from build123d import *

# Parameters (mm, degrees)
SKETCH_1_R              = 12
EXTRUDE_1_DEPTH         = 12
DELETE_BODY_1_OUTLINE_R = 5
DELETE_BODY_1_DEPTH     = 12
EXTRUDE_START           = -1
SKETCH_2_R              = 12
EXTRUDE_2_DEPTH         = 1
SKETCH_3_W              = 2
SKETCH_3_H              = 13
SKETCH_5_W              = 34.262916627
SKETCH_5_H              = 20.154656839
CUT_EXTRUDE_3_DEPTH     = 24.151673806
SKETCH_6_R              = 1.25
EXTRUDE_4_DEPTH         = 2
SKETCH_7_R              = 4
EXTRUDE_5_DEPTH         = 2


# Read off the part's stored shape, not the designer's step: the other step, the delete body step
with BuildPart() as part:
    # Sketch 1 → Extrude 1 (new body)
    with BuildSketch(Plane.XY):
        Circle(SKETCH_1_R)
    extrude(amount=EXTRUDE_1_DEPTH)

    # Other 1 outline → Other 1 (revolve, cut)
    with BuildSketch(Plane.XZ):
        with BuildLine():
            Line((12, 12), (4, 12))
            Line((4, 12), (4, 8))
            Line((4, 8), (5, 8))
            Line((5, 8), (5, 4))
            Line((5, 4), (4, 4))
            Line((4, 4), (4, 0))
            Line((4, 0), (12, 0))
            Line((12, 0), (12, 1))
            ThreePointArc((12, 1), (7, 6), (12, 11))
            Line((12, 11), (12, 12))
        make_face()
    revolve(axis=Axis((0, 0, 0), (0, 0, 1)), mode=Mode.SUBTRACT)

    # Delete Body 1 outline → Delete Body 1 (cut)
    with BuildSketch(Plane.XY):
        Circle(DELETE_BODY_1_OUTLINE_R)
    extrude(amount=DELETE_BODY_1_DEPTH, mode=Mode.SUBTRACT)



with BuildPart() as body_2:
    # Sketch 2 → Extrude 2 (new body)
    with BuildSketch(Plane.XY.offset(EXTRUDE_START)):
        with Locations(Location((0, 0, 0), (0, 0, 270))):
            Circle(SKETCH_2_R)
    extrude(amount=EXTRUDE_2_DEPTH)


with BuildPart() as part_1:
    add(part.part)

    add(body_2.part)  # Revolve 1 merges body 2
    # Sketch 3 → Revolve 1 (revolve)
    with BuildSketch(Plane(origin=(0, 0, 0), x_dir=(1, 0, 0), z_dir=(0, 1, 0))):
        with Locations((-13, -5.5)):
            Rectangle(SKETCH_3_W, SKETCH_3_H)
    revolve(axis=Axis((0, 0, 0), (0, 0, 1)))

    # Sketch 5 → Cut-Extrude 3 (cut, through all)
    with BuildSketch(Plane(origin=(0, 0, 0), x_dir=(1, 0, 0), z_dir=(0, 1, 0))):
        with Locations((0.6382308, -6.140467699)):
            Rectangle(SKETCH_5_W, SKETCH_5_H)
    extrude(amount=-CUT_EXTRUDE_3_DEPTH, mode=Mode.SUBTRACT)

    # Sketch 6 → Extrude 4 (add)
    with BuildSketch(Plane.XZ):
        with Locations(Location((-10.1, 6, 0), (0, 0, 90))):
            Circle(SKETCH_6_R)
        with Locations(Location((10.1, 6, 0), (0, 0, 90))):
            Circle(SKETCH_6_R)
    extrude(amount=EXTRUDE_4_DEPTH)

    # Sketch 7 → Extrude 5 (add)
    with BuildSketch(Plane(origin=(0, 0, -1), x_dir=(-1, 0, 0), z_dir=(0, 0, -1))):
        Circle(SKETCH_7_R)
    extrude(amount=-EXTRUDE_5_DEPTH)


solid = part_1.part
Could you check a few things on this model? Use its own coordinates, in mm. A direction names the side the tool comes from. Coordinates: 2 decimals unless noted, no trailing zeros. Loops run counter-clockwise (first coordinate to the right, second up) from the corner with the lowest first, then second, coordinate; pieces in that order, holes last.
1. Imagine slicing it at D-D (z = 4). Please give me the cut outline in (x, y), and give its area (3 significant figures).
2. For P1, Ø3, axis at x = 9.5, z = 3, coming from the -Y side; P2, Ø4, axis at x = 2.5, z = 8.5, coming from the -Y side; P3, Ø0.8, axis at x = 10, z = 5.5, coming from the -Y side, each with a flat end and sliding along its axis, tell me the tip position at first contact or that it passes through.
3. Imagine slicing it at A-A (z = 0.5). Please give me the cut outline in (x, y).
4. I need wall thicknesses on L1, parallel to Z at x = 8.25, y = 5; L2, parallel to Z at x = -9, y = 2.5; L3, parallel to X at y = 1, z = 5. Which ranges of each line are inside material? Lowest first, please.
5. For faces 1 (the face through (-10, -2, 6)), 2 (the face through (0, 0, 1)), 3 (the face through (0.264, 11.997, 0.493)), 4 (the face through (-8.88, -0.99, 5.73)), which set-ups out of +Z, -Z, +X, -X, +Y, -Y let a thin tool reach every point of the face, with its end or its side?
6. Imagine slicing it at C-C (x = 0). Please give me the cut outline in (y, z), and give its area (3 significant figures).
7. We'd pull the mould along Y, two halves only. Please class faces 5 (the face through (11, 0, 4)), 6 (the face through (0, 5, -1)), 7 (the face through (0, 6, 0)), 8 (the face through (0.867, -3.905, 0.208)): released by +Y, released by -Y, zero draft, split by the parting line, or undercut.
8. Imagine slicing it at B-B (z = 6). Please give me the cut outline in (x, y), and give its area (3 significant figures).
Computed values:
1. outline: (-14, 0) - (-7.42, 0) arc R7.42 cw to (7.42, 0) - (14, 0) arc R14 ccw to start
1. area: 221 mm2
2. P1: stops at y = 0
2. P2: stops at y = 5.86
2. P3: stops at y = -2
3. outline: (-14, 0) - (-12, 0) arc R12 cw to (12, 0) - (14, 0) arc R14 ccw to start; circle Ø8 at (0, 0)
4. L1: z = -1 to 0, 1.59 to 10.41
4. L2: z = -1 to 0, 1.77 to 10.23
4. L3: x = -13.96 to -7.03, 7.03 to 13.96
5. face 1: +Z, -Z, +X, -X, -Y
5. face 2: +Z, -Y
5. face 3: none
5. face 4: -Y
6. outline: (-4, -1) - (14, -1) - (14, 12) - (12, 12) - (12, 11) arc R5 ccw to (12, 1) - (12, 0) - (4, 0) - (4, 1) - (-4, 1) - close
6. area: 89.3 mm2
7. face 5: released by -Y
7. face 6: zero draft
7. face 7: undercut
7. face 8: undercut
8. outline: (-14, 0) - (-11.35, 0) - (-11.35, -2) - (-8.85, -2) - (-8.85, 0) - (-7, 0) arc R7 cw to (7, 0) - (8.85, 0) - (8.85, -2) - (11.35, -2) - (11.35, 0) - (14, 0) arc R14 ccw to start
8. area: 241 mm2
